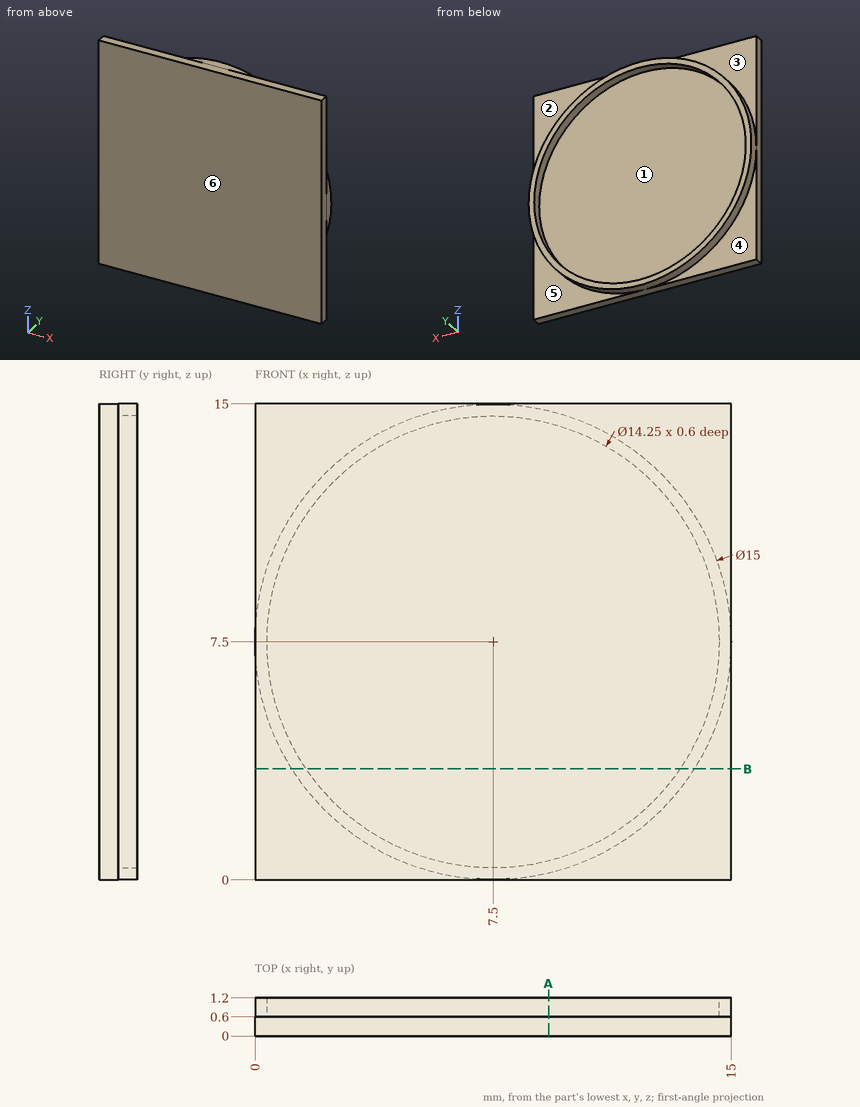
Could you check a few things on this drawing? It's one solid part, dimensions in mm from its lowest x, y, z. A direction names the side the tool comes from. Give positions to 0.01 mm unless a question says otherwise; leave off trailing zeros. Order: outer loops, then holes, each group sorted by start corner. A loop starts at its lowest first (then second) coordinate and runs counter-clockwise, first axis right, second up. Notation, with made-up numbers: (12.25, 41.25) - (27.25, 41.25) arc R28 ccw to (27.25, 76.25) - close; hole circle Ø9 at (-31, -16.75). An arc over 180 degrees is marked (long way). One line per item, written item: value. Start each with the question number.
1. If I drill on probe 1 along Z at (x, y) = (7.5, 0.9) (3 decimals); probe 2 along Y at (x, z) = (7.5, 1), over which ranges is the centre line in solid material (lowest first)?
2. Thinking about a two-plate mould opening in Z: for the marked faces 1 and 2, which applies, +Z half, -Z half, draft (parallel to the pull), parting line (faces both ways), or undercut?
3. Imagine slicing it at B-B on z = 3.5. List the corners of the cut face in (x, y) for me, plus the area to 3 significant figures.
4. Imagine slicing it at A-A on x = 9.25. List the corners of the cut face in (y, z) for me.
5. For the marked faces 3, 4, 5 and 6, which set-ups out of +Z, -Z, +X, -X, +Y, -Y let a thin tool reach every point of the face, with its end or its side?
6. For P1, Ø1, axis at x = 2, z = 8, coming from the +Y side, with a flat end and sliding along its axis, tell me the tip position at first contact or that it passes through.
Values:
1. probe 1: 0 to 0.375, 14.625 to 15
1. probe 2: 0 to 0.6
2. face 1: undercut
2. face 2: draft
3. outline: (0, 0) - (15, 0) - (15, 0.6) - (13.84, 0.6) - (13.84, 1.2) - (13.4, 1.2) - (13.4, 0.6) - (1.6, 0.6) - (1.6, 1.2) - (1.16, 1.2) - (1.16, 0.6) - (0, 0.6) - close
3. area: 9.54 mm²
4. outline: (0, 0) - (0.6, 0) - (0.6, 0.21) - (1.2, 0.21) - (1.2, 0.59) - (0.6, 0.59) - (0.6, 14.41) - (1.2, 14.41) - (1.2, 14.79) - (0.6, 14.79) - (0.6, 15) - (0, 15) - close
5. face 3: +Z, -X, +Y
5. face 4: -Z, -X, +Y
5. face 5: -Z, +X, +Y
5. face 6: +Z, -Z, +X, -X, -Y
6. P1: y = 0.6
